For this review, take the finished solid that the model builds, in its own axes (mm). Coordinates: 2 decimals unless noted, no trailing zeros. Write each loop counter-clockwise with the first axis right and the second up, starting at its lowest first coordinate (ties: lowest second). Pieces come first, ordered by that corner, then holes.
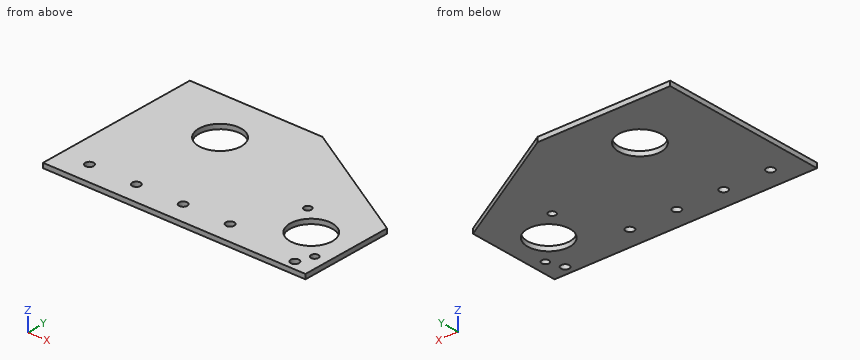
```python
from build123d import *

# Parameters (mm, degrees)
SKETCH1_W              = 177.8
SKETCH1_H              = 114.3
BOSS_EXTRUDE1_DEPTH    = 3.175
SKETCH2_R              = 14.2875
CUT_EXTRUDE1_DEPTH     = 3.175
F_10_CLEARANCE_HOLE1_D = 5.6134
SKETCH5_R              = 14.2875
SKETCH5_R_2            = 2.4892
CUT_EXTRUDE2_DEPTH     = 4.175
CHAMFER1_SIZE          = 50.8
CHAMFER1_SIZE2         = 87.988181024
F_10_CLEARANCE_HOLE2_D = 5.6134


with BuildPart() as part:
    # Sketch1 → Boss-Extrude1 (new body)
    with BuildSketch(Plane.XY):
        Rectangle(SKETCH1_W, SKETCH1_H)
    extrude(amount=BOSS_EXTRUDE1_DEPTH)

    # Sketch2 → Cut-Extrude1 (cut)
    with BuildSketch(Plane.XY.offset(3.175)):
        with Locations((-38.1, 22.352)):
            Circle(SKETCH2_R)
    extrude(amount=-CUT_EXTRUDE1_DEPTH, mode=Mode.SUBTRACT)

    # #10 Clearance Hole1 (through all)
    with Locations(Plane.XY.offset(3.175)):
        with Locations((-69.85, -42.8625), (-38.1, -42.8625), (-6.35, -42.8625), (25.4, -42.8625)):
            Hole(F_10_CLEARANCE_HOLE1_D / 2)

    # Sketch5 → Cut-Extrude2 (cut, through all)
    with BuildSketch(Plane.XY.offset(3.175)):
        with Locations((62.443181743, -22.225)):
            Circle(SKETCH5_R)
        with Locations((44.482669501, -4.264487758)):
            Circle(SKETCH5_R_2)
        with Locations((80.403693985, -40.185512242)):
            Circle(SKETCH5_R_2)
    extrude(amount=-CUT_EXTRUDE2_DEPTH, mode=Mode.SUBTRACT)

    # Chamfer1
    chamfer1_edges = [part.edges().sort_by_distance(p)[0] for p in [
        (88.9, 57.15, 1.5875),
    ]]
    chamfer1_side = [part.faces().sort_by_distance(p)[0] for p in [
        (88.9, 0, 1.5875),
    ]]
    chamfer(chamfer1_edges, length=CHAMFER1_SIZE, length2=CHAMFER1_SIZE2, reference=chamfer1_side[0])

    # #10 Clearance Hole2 (through all)
    with Locations(Plane(origin=(0, 0, 0), x_dir=(-1, 0, 0), z_dir=(0, 0, -1))):
        with Locations((-76.2, -50.8)):
            Hole(F_10_CLEARANCE_HOLE2_D / 2)


solid = part.part
```
1) Clearance check with flat-ended pins moving along their axes: P1, Ø7.5, axis at x = -6.35, y = -42.86, coming from the -Z side; P2, Ø4.5, axis at x = -38.1, y = -42.86, coming from the -Z side; P3, Ø1, axis at x = 55.5, z = 0.5, coming from the +Y side; P4, Ø1, axis at x = 27, z = 1.5, coming from the +Y side. State where each tip first meets the part, or that it passes through.
2) Consider section B-B (y = -50.8). Give the boundary of the cut face in (x, z) (3 decimals), then the cut area to 3 significant figures.
3) For L1, parallel to Y at x = -38.1, z = 2.2; L2, parallel to X at y = -43, z = 0.75; L3, parallel to X at y = -13, z = 1.9, list the stretches that pass through material, from the lowest coordinate up.
4) Consider section A-A (x = -38.1). Count the separate pieces of the cut face and the enclosed holes in it, then the cut area to 3 significant figures.
5) Consider section C-C (x = -69.85). Give the boundary of the cut face in (y, z) (3 decimals).
Results:
1. P1: stops at z = 0
1. P2: passes through
1. P3: stops at y = 25.92
1. P4: stops at y = 42.38
2. outline: (-88.9, 0) - (73.393, 0) - (73.393, 3.175) - (-88.9, 3.175) - close; (79.007, 0) - (88.9, 0) - (88.9, 3.175) - (79.007, 3.175) - close
2. area: 547 mm2
3. L1: y = -57.15 to -45.67, -40.06 to 8.06, 36.64 to 57.15
3. L2: x = -88.9 to -72.65, -67.05 to -40.9, -35.3 to -9.15, -3.55 to 22.6, 28.2 to 88.9
3. L3: x = -88.9 to 51.53, 73.35 to 88.9
4. separate pieces: 3
4. enclosed holes: 0
4. area: 254 mm2
5. outline: (-57.15, 0) - (-45.669, 0) - (-45.669, 3.175) - (-57.15, 3.175) - close; (-40.056, 0) - (57.15, 0) - (57.15, 3.175) - (-40.056, 3.175) - close
